Source: CAD feature listing. Evaluate the final solid. Frame: model axes, mm. A direction names the side the tool comes from. Round coordinates to 2 decimals unless told otherwise and drop trailing zeros. Write each loop counter-clockwise with the first axis right and the second up, starting at its lowest first coordinate (ties: lowest second). Pieces come first, ordered by that corner, then holes. Notation, with made-up numbers: (4.5, 1.25) -> (53.5, 1.25) arc R23 cw to (53.5, 10.25) -> close; hole circle Ø7 at (-40, 82.25). An arc over 180 degrees is marked (long way). Put each result on its own line as item: value.
```python
from build123d import *
from OCP.BRepFilletAPI import BRepFilletAPI_MakeChamfer

# Parameters (mm, degrees)
SKETCH1_R               = 23.7
SKETCH1_R_2             = 18.7
BOSS_EXTRUDE1_DEPTH     = 48
BOSS_EXTRUDE2_START     = 5
SKETCH1_3_R             = 23.7
SKETCH1_3_R_2           = 18.7
SKETCH1_3_R_3           = 15.5
SKETCH1_3_R_4           = 6.5
BOSS_EXTRUDE2_DEPTH     = 5
M3_CLEARANCE_HOLE1_D    = 3.4
CIRPATTERN1_COUNT       = 6
BOSS_EXTRUDE3_DEPTH     = 38.1
F_1_4_CLEARANCE_HOLE1_D = 6.7564
SKETCH9_R               = 5.715
CUT_EXTRUDE1_DEPTH      = 89.454226705
CHAMFER1_SIZE           = 5
CHAMFER1_SIZE2          = 3.549039071


with BuildPart() as part:
    # Sketch1 → Boss-Extrude1 (new body)
    with BuildSketch(Plane.XY):
        Circle(SKETCH1_R)
        Circle(SKETCH1_R_2, mode=Mode.SUBTRACT)
    extrude(amount=-BOSS_EXTRUDE1_DEPTH)

    # Sketch1_3 → Boss-Extrude2 (add)
    # profile 1 of 3: a face of its own
    with BuildSketch(Plane.XY.offset(BOSS_EXTRUDE2_START)):
        Circle(SKETCH1_3_R)
        Circle(SKETCH1_3_R_2, mode=Mode.SUBTRACT)
    # profile 2 of 3: a face of its own
    with BuildSketch(Plane.XY.offset(BOSS_EXTRUDE2_START)):
        Circle(SKETCH1_3_R_2)
        Circle(SKETCH1_3_R_3, mode=Mode.SUBTRACT)
    # profile 3 of 3: a face of its own
    with BuildSketch(Plane.XY.offset(BOSS_EXTRUDE2_START)):
        Circle(SKETCH1_3_R_3)
        with Locations((0, 7.5)):
            Circle(SKETCH1_3_R_4, mode=Mode.SUBTRACT)
    extrude(amount=-BOSS_EXTRUDE2_DEPTH)

    # M3 Clearance Hole1 (through all)
    with Locations(Plane.XY.offset(5)):
        with Locations((-15.5, 0)):
            m3_clearance_hole1 = Hole(M3_CLEARANCE_HOLE1_D / 2)

    # CirPattern1: M3 Clearance Hole1 ×6 about axis
    cirpattern1_axis = Axis((0, 0, 0), (0, 0, 1))
    for i in range(1, CIRPATTERN1_COUNT):
        add(m3_clearance_hole1.rotate(cirpattern1_axis, i * 360 / CIRPATTERN1_COUNT), mode=Mode.SUBTRACT)

    # Sketch5 → Boss-Extrude3 (add)
    with BuildSketch(Plane.XY.offset(5)):
        with BuildLine():
            Line((56.111141692, 30), (-56.111141692, 30))
            Line((-56.111141692, 30), (-18.155253302, -15.23406635))
            ThreePointArc((-18.155253302, -15.23406635), (-8.105877397, 22.270715113), (23.7, 0))
            ThreePointArc((23.7, 0), (22.270715113, -8.105877397), (18.155253302, -15.23406635))
            Line((18.155253302, -15.23406635), (56.111141692, 30))
        make_face()
    extrude(amount=-BOSS_EXTRUDE3_DEPTH)

    # 1_4 Clearance Hole1 (through all)
    with Locations(Plane(origin=(0, 30, 0), x_dir=(1, 0, 0), z_dir=(0, 1, 0))):
        with Locations((-45, 20.4), (45, 20.4)):
            Hole(F_1_4_CLEARANCE_HOLE1_D / 2)

    # Sketch9 → Cut-Extrude1 (cut, through all)
    with BuildSketch(Plane(origin=(0, 25, 0), x_dir=(1, 0, 0), z_dir=(0, 1, 0))):
        with Locations(Location((-45, 20.4, 0), (0, 0, 180))):
            Circle(SKETCH9_R)
        with Locations(Location((45, 20.4, 0), (0, 0, 180))):
            Circle(SKETCH9_R)
    extrude(amount=-CUT_EXTRUDE1_DEPTH, mode=Mode.SUBTRACT)

    # Chamfer1: one chamfer whose edges measure the first distance from different faces: ONE call of the kernel's chamfer builder (chamfer() names one face for all edges)
    chamfer1_edges_1 = [part.edges().sort_by_distance(p)[0] for p in [
        (56.111141692, 30, -14.05),
    ]]
    chamfer1_side_1 = [part.faces().sort_by_distance(p)[0] for p in [
        (36.532384477, 6.666945749, -13.565030067),
    ]]
    chamfer1_edges_2 = [part.edges().sort_by_distance(p)[0] for p in [
        (-56.111141692, 30, -14.05),
    ]]
    chamfer1_side_2 = [part.faces().sort_by_distance(p)[0] for p in [
        (-36.532384477, 6.666945749, -13.565030067),
    ]]
    chamfer1 = BRepFilletAPI_MakeChamfer(part.part.solid().wrapped)
    for e in chamfer1_edges_1:
        chamfer1.Add(CHAMFER1_SIZE, CHAMFER1_SIZE2, e.wrapped, chamfer1_side_1[0].wrapped)  # the first distance lies on this face
    for e in chamfer1_edges_2:
        chamfer1.Add(CHAMFER1_SIZE, CHAMFER1_SIZE2, e.wrapped, chamfer1_side_2[0].wrapped)  # the first distance lies on this face
    add(Compound.cast(chamfer1.Shape()), mode=Mode.REPLACE)


solid = part.part
```
Q1. Cut plane D-D on y = 22. Output: boundary loops of the cut face in (x, z) (3 decimals).
Ans:
outline: (-49.398, -33.1) -> (-8.814, -33.1) -> (-8.814, -48) -> (8.814, -48) -> (8.814, -33.1) -> (49.398, -33.1) -> (49.398, -24.049) arc R5.715 cw (long way) to (49.398, -16.751) -> (49.398, 5) -> (-49.398, 5) -> (-49.398, -16.751) arc R5.715 cw (long way) to (-49.398, -24.049) -> close
Q2. Cut plane B-B on x = 15.5. Output: boundary loops of the cut face in (y, z), and give its area (3 significant figures).
Ans:
outline: (-17.93, -48) -> (-10.46, -48) -> (-10.46, 0) -> (-1.7, 0) -> (-1.7, 5) -> (-17.93, 5) -> close; (1.7, 0) -> (10.46, 0) -> (10.46, -48) -> (17.93, -48) -> (17.93, -33.1) -> (30, -33.1) -> (30, 5) -> (1.7, 5) -> close
area: 1,340 mm^2
Q3. Reachability of faces 4 (the cylindrical face through (-39.29, 19.14, -20.15)), 5 (the cylindrical face through (-17.07, -0.65, 2.47)), 6 (the cylindrical face through (-4.054, -18.255, -23.664)) from +Z, -Z, +X, -X, +Y, -Y: full face, straight path, thin tool, end or side. Return the list, or none.
Ans:
face 4: -Y
face 5: +Z, -Z
face 6: -Z
Q4. Cut plane A-A on z = -20.4. Output: boundary loops of the cut face in (x, y) (3 decimals), and give its area (3 significant figures).
Ans:
outline: (-52.897, 26.17) -> (-50.715, 23.569) -> (-50.715, 25) -> (-48.378, 25) -> (-48.378, 30) -> (-52.562, 30) -> close; (-41.622, 25) -> (-39.285, 25) -> (-39.285, 9.947) -> (-18.155, -15.234) arc R23.7 ccw to (18.155, -15.234) -> (39.285, 9.947) -> (39.285, 25) -> (41.622, 25) -> (41.622, 30) -> (-41.622, 30) -> close; (48.378, 25) -> (50.715, 25) -> (50.715, 23.569) -> (52.897, 26.17) -> (52.562, 30) -> (48.378, 30) -> close; hole circle Ø37.4 at (0, 0)
area: 2,200 mm^2
Q5. Cut plane C-C on z = -2. Output: boundary loops of the cut face in (x, y), and give its area (3 significant figures).
Ans:
outline: (-52.9, 26.17) -> (-18.16, -15.23) arc R23.7 ccw to (18.16, -15.23) -> (52.9, 26.17) -> (52.56, 30) -> (-52.56, 30) -> close; hole circle Ø37.4 at (0, 0)
area: 2,460 mm^2
Q6. Draft query along Y for faces 1 (the flat face through (42.5, 25, -22.9)), 2 (the flat face through (-1, 15, 5)), 3 (the cylindrical face through (-6.966, 14.932, 2.465)). Return one class per face: +Y half, -Y half, draft (parallel to the pull), parting line (faces both ways), or undercut.
Ans:
face 1: -Y half
face 2: draft
face 3: undercut
Q7. Material intervals for line 1 (X direction, y = 28.15, z = -20.4); line 2 (Z direction, x = 2, y = 26); line 3 (X direction, y = 1, z = -16.5), sorted ascending. Write a range as [from, to].
Ans:
line 1: x = [-52.72, -48.38], [-41.62, 41.62], [48.38, 52.72]
line 2: z = [-33.1, 5]
line 3: x = [-31.78, -18.67], [18.67, 31.78]
Q8. Pin query (flat end, axial travel): pin 1 (6 mm diameter, centred on y = -14.5, z = -15, fed in from +X); pin 2 (4.5 mm diameter, centred on x = 7.75, y = 13.42, fed in from -Z); pin 3 (4 mm diameter, centred on x = 45, z = -20.4, fed in from -Y); pin 4 (3 mm diameter, centred on y = 24, z = -25.5, fed in from -X). Return the tip coordinate at first contact, or that it passes through.
Ans:
pin 1: stops at x = 21.29
pin 2: stops at z = 0
pin 3: passes through
pin 4: stops at x = -52.34
